Source: CAD feature listing. Evaluate the final solid. Frame: model axes, mm. A direction names the side the tool comes from. Round coordinates to 2 decimals unless told otherwise and drop trailing zeros. Write each loop counter-clockwise with the first axis right and the second up, starting at its lowest first coordinate (ties: lowest second). Pieces come first, ordered by that corner, then holes. Notation, with made-up numbers: M 14.25,8.25 L 49.25,8.25 A26 cw 49.25,36.25 Z; hole C -32,82.5 d2. An arc over 180 degrees is marked long. Answer in a Markdown table with one row per item. Add a question column.
Item 1: Cut plane B-B on z = 50. Return loops of the section in (x, y).
Item 2: Cut plane A-A on x = 0. Return loops of the section in (y, z).
Item 3: Mould query, pull axis X, two halves, no side actions, for faces 1 (the face through (70.545, 0, 30)), 2 (the face through (0, 45, 40)), 3 (the face through (-70.545, 0, 30)), 4 (the face through (61.664, 0, 30)). Classes: released by +X, released by -X, zero draft, split by the parting line, or undercut.
Item 4: Contact query for flat-ended pins moving along their axis: pin 1 (3 mm diameter, centred on x = -18.5, z = 102.5, fed in from +Y); pin 2 (10 mm diameter, centred on y = 20.5, z = 35, fed in from -X); pin 3 (4.5 mm diameter, centred on x = -67.5, z = 28.5, fed in from +Y); pin 4 (6 mm diameter, centred on x = 37, y = 22.5, fed in from -Z). Output: stop coordinate, or through.
Item 5: Material intervals for probe 1 along X at (y, z) = (1, 30.5); probe 2 along X at (y, z) = (6, 32); probe 3 along Y at (x, z) = (4.5, 49), sorted ascending.
Item 6: Set-up query: faces 5 (the face through (-67.156, 11.486, 26.662)), 6 (the face through (0, 40, 50)), 7 (the face through (-63.916, 0.14, 33.863)), 8 (the face through (0, -40, 50)). Return all of +Z, -Z, +X, -X, +Y, -Y with unobstructed straight access to the full face (end or side cutting, diameter ignored); none if empty.
from build123d import *

# Parameters (mm, degrees)
IZIM1_R                     = 50
Y_KSEKLIK_EKSTR_ZYON1_DEPTH = 150
PAH1_SIZE                   = 30
PAH1_SIZE2                  = 10.919107028
KES_EKSTR_ZYON1_DEPTH       = 50
S_P_R1_PROFILE_R            = 3.5
KES_EKSTR_ZYON2_START       = -40
IZIM20_R                    = 10
KES_EKSTR_ZYON2_DEPTH       = 100
Y_KSEKLIK_EKSTR_ZYON2_DEPTH = 10


with BuildPart() as part:
    # Çizim1 → Yükseklik-Ekstrüzyon1 (new body)
    with BuildSketch(Plane.XY):
        Circle(IZIM1_R)
    extrude(amount=Y_KSEKLIK_EKSTR_ZYON1_DEPTH)

    # Pah1
    pah1_edges = [part.edges().sort_by_distance(p)[0] for p in [
        (-50, 0, 150),
    ]]
    pah1_side = [part.faces().sort_by_distance(p)[0] for p in [
        (-50, 0, 75),
    ]]
    chamfer(pah1_edges, length=PAH1_SIZE, length2=PAH1_SIZE2, reference=pah1_side[0])

    # Çizim5 → Kes-Ekstrüzyon1 (cut, symmetric)
    with BuildSketch(Plane(origin=(0, 0, 0), x_dir=(1, 0, 0), z_dir=(0, 1, 0))):
        Polygon((-50, -120), (-120.002601454, -158.048405528), (-22.959282712, -158.048405528), align=None)
        Polygon((22.959282712, -158.048405528), (50, -120), (120.002601454, -158.048405528), align=None)
    extrude(amount=KES_EKSTR_ZYON1_DEPTH, both=True, mode=Mode.SUBTRACT)

    # Süpür1: sweep along a path in Çizim6
    with BuildLine(Plane.XY.offset(30)) as s_p_r1_path:
        Line((-44.301038276, -19.710381189), (-59.325338364, -19.710381189))
        ThreePointArc((-59.325338364, -19.710381189), (-64.118952606, -17.724801158), (-66.104532637, -12.931186916))
        Line((-66.104532637, -12.931186916), (-66.104532637, 12.931186916))
        ThreePointArc((-66.104532637, 12.931186916), (-64.118952606, 17.724801158), (-59.325338364, 19.710381189))
        Line((-59.325338364, 19.710381189), (-44.301038276, 19.710381189))
    # Süpür1 profile (on start of the path) → Süpür1 (sweep)
    with BuildSketch(Plane(origin=(-44.301038276, -19.710381189, 30), x_dir=(0, 0, -1), z_dir=(-1, 0, 0))):
        Circle(S_P_R1_PROFILE_R)
    s_p_r1 = sweep(path=s_p_r1_path.line)

    # Aynalama1: Süpür1 across plane
    add(s_p_r1.mirror(Plane(origin=(0, 0, 0), x_dir=(0, 0, 1), z_dir=(1, 0, 0))))

    # Çizim20 → Kes-Ekstrüzyon2 (cut)
    with BuildSketch(Plane(origin=(0, 0, 0), x_dir=(1, 0, 0), z_dir=(0, 1, 0)).offset(KES_EKSTR_ZYON2_START)):
        with Locations(Location((0, -50, 0), (0, 0, 270))):
            Circle(IZIM20_R)
    kes_ekstr_zyon2 = extrude(amount=-KES_EKSTR_ZYON2_DEPTH, mode=Mode.SUBTRACT)

    # Aynalama2: Kes-Ekstrüzyon2 across plane
    add(kes_ekstr_zyon2.mirror(Plane.ZX), mode=Mode.SUBTRACT)

    # Çizim21 → Yükseklik-Ekstrüzyon2 (add, symmetric)
    with BuildSketch(Plane(origin=(0, 0, 0), x_dir=(1, 0, 0), z_dir=(0, 1, 0))):
        Polygon((-66.104532637, -35.126982438), (-61.664435601, -32.563491219), (-61.664435601, -27.436508781), (-66.104532637, -24.873017562), (-70.544629673, -27.436508781), (-70.544629673, -32.563491219), align=None)
    y_kseklik_ekstr_zyon2 = extrude(amount=Y_KSEKLIK_EKSTR_ZYON2_DEPTH, both=True)

    # Aynalama3: Yükseklik-Ekstrüzyon2 across plane
    add(y_kseklik_ekstr_zyon2.mirror(Plane(origin=(0, 0, 0), x_dir=(0, 0, 1), z_dir=(1, 0, 0))))


solid = part.part
Results below:
| question | item | result |
|---|---|---|
| 1 | outline | M -10,-48.99 L -10,-40 L 10,-40 L 10,-48.99 A50 ccw 10,48.99 L 10,40 L -10,40 L -10,48.99 A50 ccw Z |
| 2 | outline | M -50,0 L 50,0 L 50,40 L 40,40 L 40,60 L 50,60 L 50,120 L 39.08,150 L -39.08,150 L -50,120 L -50,60 L -40,60 L -40,40 L -50,40 Z |
| 3 | face 1 | released by +X |
| 3 | face 2 | undercut |
| 3 | face 3 | released by -X |
| 3 | face 4 | undercut |
| 4 | pin 1 | y = 47.02 |
| 4 | pin 2 | x = -68.43 |
| 4 | pin 3 | y = 21.14 |
| 4 | pin 4 | z = 0 |
| 5 | probe 1 | -70.54 to -61.66, -49.99 to 49.99, 61.66 to 70.54 |
| 5 | probe 2 | -70.54 to -61.66, -49.64 to 49.64, 61.66 to 70.54 |
| 5 | probe 3 | -40 to 40 |
| 6 | face 5 | none |
| 6 | face 6 | +Y |
| 6 | face 7 | +Z |
| 6 | face 8 | -Y |
